```python
from build123d import *

# Parameters (mm, degrees)
SKETCH3_W                           = 101.6
SKETCH3_H                           = 11.1125
BOSS_EXTRUDE1_DEPTH                 = 50.8
BASEBORDERRADIUSSKETCH_OUTSIDE_W    = 132.41
BASEBORDERRADIUSSKETCH_OUTSIDE_H    = 132.41
BASEBORDERRADIUSSKETCH_OUTSIDE_W_2  = 95.25
BASEBORDERRADIUSSKETCH_OUTSIDE_H_2  = 95.25
BASEBORDERRADIUSCUT_EXTRUDE_DEPTH   = 73.57931249
BUMPER_6_32_TAPPED_HOLE_D           = 4.3053
BUMPER_6_32_TAPPED_HOLE_CBORE_D     = 7.9375
BUMPER_6_32_TAPPED_HOLE_CBORE_DEPTH = 5.3848
BUMPERTHREADLPATTERN_COUNT          = 2
BUMPERTHREADLPATTERN_PITCH          = 76.2
BUMPERTHREADLPATTERN_COUNT_DIR2     = 2
BUMPERTHREADLPATTERN_PITCH_DIR2     = 76.2


with BuildPart() as part:
    # Sketch3 → Boss-Extrude1 (new, symmetric)
    with BuildSketch(Plane.XY):
        Rectangle(SKETCH3_W, SKETCH3_H)
    extrude(amount=BOSS_EXTRUDE1_DEPTH, both=True)

    # FacingTopSurfaceCut
    split(bisect_by=Plane(origin=(0, 5.159375, 0), x_dir=(1, 0, 0), z_dir=(0, 1, 0)), keep=Keep.BOTTOM)

    # FacingBottomSurfaceCut
    split(bisect_by=Plane(origin=(0, -5.159375, 0), x_dir=(-1, 0, 0), z_dir=(0, -1, 0)), keep=Keep.BOTTOM)

    # BaseBorderRadiusSketch outside → BaseBorderRadiusCut-Extrude (cut, through all)
    with BuildSketch(Plane(origin=(0, 5.159375, 0), x_dir=(1, 0, 0), z_dir=(0, 1, 0))):
        Rectangle(BASEBORDERRADIUSSKETCH_OUTSIDE_W, BASEBORDERRADIUSSKETCH_OUTSIDE_H)
        Rectangle(BASEBORDERRADIUSSKETCH_OUTSIDE_W_2, BASEBORDERRADIUSSKETCH_OUTSIDE_H_2, mode=Mode.SUBTRACT)
    extrude(amount=-BASEBORDERRADIUSCUT_EXTRUDE_DEPTH, mode=Mode.SUBTRACT)

    # Bumper#6-32 Tapped Hole (through all)
    with Locations(Plane(origin=(-38.1, -5.159375, 38.1), x_dir=(0, 0, -1), z_dir=(0, -1, 0))):
        with Locations((0, 0), (25.4, 16.102954744), (25.4, 60.097045256), (63.5, 38.1)):
            bumper_6_32_tapped_hole = CounterBoreHole(BUMPER_6_32_TAPPED_HOLE_D / 2, BUMPER_6_32_TAPPED_HOLE_CBORE_D / 2, BUMPER_6_32_TAPPED_HOLE_CBORE_DEPTH)

    # BumperThreadLPattern: Bumper_6-32 Tapped Hole 2 × 2
    with Locations(*[(j * BUMPERTHREADLPATTERN_PITCH_DIR2, 0, -i * BUMPERTHREADLPATTERN_PITCH) for i in range(BUMPERTHREADLPATTERN_COUNT) for j in range(BUMPERTHREADLPATTERN_COUNT_DIR2) if (i, j) != (0, 0)]):
        add(bumper_6_32_tapped_hole, mode=Mode.SUBTRACT)


solid = part.part
```
Design review of the part built by this model. Coordinates are the model's own, in mm. A direction names the side the tool comes from. Give positions to 0.01 mm unless a question says otherwise; leave off trailing zeros. Order: outer loops, then holes, each group sorted by start corner. A loop starts at its lowest first (then second) coordinate and runs counter-clockwise, first axis right, second up. Notation, with made-up numbers: (0.5, 66) - (49.5, 66) arc R14 ccw to (49.5, 84) - close; hole circle Ø11 at (-12, 89). An arc over 180 degrees is marked (long way). Use a Markdown table: item, result. Add a question column.
(1) Add section B-B on z = 12.7. Give the boundary of the cut face in (x, y) (3 decimals), then the cut area to 3 significant figures.
(2) Machinability: for faces 4 (the face through (19.896, 2.727, 12.233)), 5 (the face through (36, 0.225, -40)), which of the approach directions +Z, -Z, +X, -X, +Y, -Y give a long, thin tool a straight path to every point of the face, cutting with its end or side? Answer none if there is none.
(3) Mouldability with a two-part tool opening along Z and no side actions: class faces 1 (the face through (-1, 0, 47.625)), 2 (the face through (-47.625, 0, 1)), 3 (the face through (-35.966, 2.727, 37.82)) as +Z half, -Z half, draft (parallel to the pull), parting line (faces both ways), or undercut.
(4) Clearance check with flat-ended pins moving along their axes: P1, Ø3.5, axis at x = 38.1, z = 38.1, coming from the -Y side; P2, Ø4, axis at x = -22, z = 12.5, coming from the -Y side; P3, Ø7, axis at x = -22, z = 12.7, coming from the +Y side. State where each tip first meets the part, or that it passes through.
(5) Add section C-C on y = -1.5. Give the boundary of the cut face in (x, z) (1 decimal), then the cut area to 3 significant figures.
(6) Add section A-A on x = 38.1. Give the boundary of the cut face in (y, z) (3 decimals), then the cut area to 3 significant figures.
(7) Wall thickness on probe 1 along X at (y, z) = (3.15, 12.7) (3 decimals); probe 2 along X at (y, z) = (3.15, -38.1) (3 decimals); probe 3 along X at (y, z) = (-1.1, -25.4) (3 decimals): over which ranges is each line inside the solid? List them lowest first. Write a range as [from, to].
Report:
| question | item | result |
|---|---|---|
| 1 | outline | (-47.625, -5.159) - (-25.966, -5.159) - (-25.966, 0.225) - (-24.15, 0.225) - (-24.15, 5.159) - (-47.625, 5.159) - close; (-19.844, 0.225) - (-18.028, 0.225) - (-18.028, -5.159) - (18.028, -5.159) - (18.028, 0.225) - (19.844, 0.225) - (19.844, 5.159) - (-19.844, 5.159) - close; (24.15, 0.225) - (25.966, 0.225) - (25.966, -5.159) - (47.625, -5.159) - (47.625, 5.159) - (24.15, 5.159) - close |
| 1 | area | 855 mm² |
| 2 | face 4 | +Y, -Y |
| 2 | face 5 | -Y |
| 3 | face 1 | +Z half |
| 3 | face 2 | draft |
| 3 | face 3 | undercut |
| 4 | P1 | passes through |
| 4 | P2 | stops at y = 0.23 |
| 4 | P3 | stops at y = 5.16 |
| 5 | outline | (-47.6, -47.6) - (47.6, -47.6) - (47.6, 47.6) - (-47.6, 47.6) - close; hole circle Ø7.9 at (-38.1, -38.1); hole circle Ø7.9 at (-38.1, 38.1); hole circle Ø7.9 at (-22, 12.7); hole circle Ø7.9 at (0, -25.4); hole circle Ø7.9 at (22, 12.7); hole circle Ø7.9 at (38.1, -38.1); hole circle Ø7.9 at (38.1, 38.1) |
| 5 | area | 8,730 mm² |
| 6 | outline | (-5.159, -47.625) - (5.159, -47.625) - (5.159, -40.253) - (0.225, -40.253) - (0.225, -42.069) - (-5.159, -42.069) - close; (-5.159, -34.131) - (0.225, -34.131) - (0.225, -35.947) - (5.159, -35.947) - (5.159, 35.947) - (0.225, 35.947) - (0.225, 34.131) - (-5.159, 34.131) - close; (-5.159, 42.069) - (0.225, 42.069) - (0.225, 40.253) - (5.159, 40.253) - (5.159, 47.625) - (-5.159, 47.625) - close |
| 6 | area | 855 mm² |
| 7 | probe 1 | x = [-47.625, -24.15], [-19.844, 19.844], [24.15, 47.625] |
| 7 | probe 2 | x = [-47.625, -40.253], [-35.947, 35.947], [40.253, 47.625] |
| 7 | probe 3 | x = [-47.625, -3.969], [3.969, 47.625] |
